CAD build for the part. Positions are in the model's coordinates, mm. Face numbers are marked on the shaded views. Round coordinates to 2 decimals unless told otherwise and drop trailing zeros. Loops run counter-clockwise (first coordinate to the right, second up) from the corner with the lowest first, then second, coordinate; pieces in that order, holes last. Notation, with made-up numbers: (-24, 24.25) - (22, 24.25) arc R18 cw to (22, 54.25) - close; hole circle Ø10 at (39, -27). An arc over 180 degrees is marked (long way). Use one line per item in the form item = value.
from build123d import *

# Parameters (mm, degrees)
IZIM1_W               = 50
IZIM1_H               = 80
TABAN_FLAN_1_DEPTH    = 10
IZIM6_R               = 4.25
KES_EKSTR_ZYON1_DEPTH = 20
RADYUS1_R             = 5


# Sheet-metal steps are written as plain solids
with BuildPart() as part:
    # Çizim1 → Taban-Flanş1 (new body)
    with BuildSketch(Plane.XY):
        Rectangle(IZIM1_W, IZIM1_H)
    extrude(amount=-TABAN_FLAN_1_DEPTH)

    # Çizim6 → Kes-Ekstrüzyon1 (cut)
    with BuildSketch(Plane.XY):
        with Locations((0, 25)):
            Circle(IZIM6_R)
        with Locations((0, -20)):
            Circle(IZIM6_R)
    extrude(amount=-KES_EKSTR_ZYON1_DEPTH, mode=Mode.SUBTRACT)

    # Radyus1
    radyus1_edges = [part.edges().sort_by_distance(p)[0] for p in [
        (25, -40, -5),
        (-25, -40, -5),
        (-25, 40, -5),
        (25, 40, -5),
    ]]
    fillet(radyus1_edges, radius=RADYUS1_R)


solid = part.part
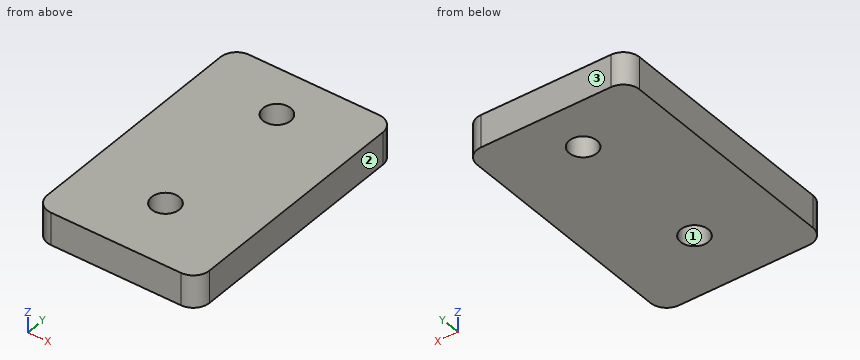
1) Two-plate mould, pull along X, no slides. Class the marked faces 1, 2 and 3: +X half, -X half, draft (parallel to the pull), parting line (faces both ways), or undercut.
Report:
face_1 = undercut
face_2 = +X half
face_3 = draft
2) Slice it at A-A (y = 25). Write the cut outline in (x, z), plus the area to 3 significant figures.
Report:
outline = (-25, -10) - (-4.25, -10) - (-4.25, 0) - (-25, 0) - close; (4.25, -10) - (25, -10) - (25, 0) - (4.25, 0) - close
area = 415 mm^2
3) Slice it at C-C (z = -4.5). Write the cut outline in (x, y), plus the area to 3 significant figures.
Report:
outline = (-25, -35) arc R5 ccw to (-20, -40) - (20, -40) arc R5 ccw to (25, -35) - (25, 35) arc R5 ccw to (20, 40) - (-20, 40) arc R5 ccw to (-25, 35) - close; hole circle Ø8.5 at (0, -20); hole circle Ø8.5 at (0, 25)
area = 3,870 mm^2
4) Slice it at B-B (x = 0). Write the cut outline in (y, z).
Report:
outline = (-40, -10) - (-24.25, -10) - (-24.25, 0) - (-40, 0) - close; (-15.75, -10) - (20.75, -10) - (20.75, 0) - (-15.75, 0) - close; (29.25, -10) - (40, -10) - (40, 0) - (29.25, 0) - close
5) Drill centre lines: probe 1 along Y at (x, z) = (0, -6.5); probe 2 along X at (y, z) = (-18.5, -3.5). Where is each one in solid material? Low to high.
Report:
probe_1 = -40 to -24.25, -15.75 to 20.75, 29.25 to 40
probe_2 = -25 to -3.98, 3.98 to 25
6) Flat gauge pin, fed straight in: pin 1 (7 mm diameter, centred on x = 0, y = 25, fed in from -Z). Where does the tip first touch, or does it go through?
Report:
pin_1 = through
